from build123d import *

# Parameters (mm, degrees)
F0_W     = 152.4
F0_H     = 76.2
F1_DEPTH = 19.05
F2_SIZE  = 19.04999
F3_W     = 152.4
F3_H     = 76.2
F4_DEPTH = 10.16
F5_T     = -2.032
F6_R     = 5.08


# Not quite as in the source:
# - a fillet or chamfer is up to 0.001 mm smaller than in the source, because OpenCascade refuses the exact size


with BuildPart() as f1:
    # F0 (on Top) → F1 (new body)
    with BuildSketch(Plane.XY):
        with Locations((-76.2, -38.1)):
            Rectangle(F0_W, F0_H)
    extrude(amount=F1_DEPTH)

    # F2 (size 19.05 in the source; OpenCascade refuses exactly that, so slightly less here)
    f2_edges = [f1.edges().sort_by_distance(p)[0] for p in [
        (0, -38.1, 19.05),
        (-76.2, 0, 19.05),
        (-152.4, -38.1, 19.05),
        (-76.2, -76.2, 19.05),
    ]]
    chamfer(f2_edges, length=F2_SIZE)

    # F3 (on face) → F4 (join)
    with BuildSketch(Plane(origin=(0, 0, 0), x_dir=(1, 0, 0), z_dir=(0, 0, -1))):
        with Locations((-76.2, 38.1)):
            Rectangle(F3_W, F3_H)
    extrude(amount=F4_DEPTH)

    # F5
    f5_openings = [f1.faces().sort_by_distance(p)[0] for p in [
        (-76.2, -38.1, -10.16),
    ]]
    offset(amount=F5_T, openings=f5_openings)

    # F6
    f6_edges = [f1.edges().sort_by_distance(p)[0] for p in [
        (0, 0, -5.08),
        (-152.4, 0, -5.08),
        (-152.4, -76.2, -5.08),
        (0, -76.2, -5.08),
    ]]
    fillet(f6_edges, radius=F6_R)


solid = f1.part
Can you work these out from the model? Positions are in its coordinate system, mm. A direction names the side the tool comes from. Give positions to 0.01 mm unless a question says otherwise; leave off trailing zeros. Order: outer loops, then holes, each group sorted by start corner. A loop starts at its lowest first (then second) coordinate and runs counter-clockwise, first axis right, second up. Notation, with made-up numbers: M -34,0.25 L -12,0.25 A15 cw -12,17.25 Z; hole C -7,-3 d5. An arc over 180 degrees is marked long. One line per item, written item: value.
Item 1: If we section it at A-A on z = -8: Write out the boundary of the cut face in (x, y).
Verdict:
outline: M -152.4,-71.12 A5.08 ccw -147.32,-76.2 L -5.08,-76.2 A5.08 ccw 0,-71.12 L 0,-5.08 A5.08 ccw -5.08,0 L -147.32,0 A5.08 ccw -152.4,-5.08 Z; hole M -150.37,-74.17 L -2.03,-74.17 L -2.03,-2.03 L -150.37,-2.03 Z
Item 2: If we section it at B-B on x = -63.5: Write out the boundary of the cut face in (y, z).
Verdict:
outline: M -76.2,-10.16 L -74.17,-10.16 L -74.17,-0.84 L -56.31,17.02 L -19.89,17.02 L -2.03,-0.84 L -2.03,-10.16 L 0,-10.16 L 0,0 L -19.05,19.05 L -57.15,19.05 L -76.2,0 Z
Item 3: For pin 1 (4 mm diameter, centred on x = -62.5, z = 9.5, fed in from +Y); pin 2 (2 mm diameter, centred on x = -33.5, z = 9, fed in from -Y); pin 3 (10 mm diameter, centred on y = -30.5, z = 9, fed in from +X), each with a flat end and sliding along its axis, tell me the tip position at first contact or that it passes through.
Verdict:
pin 1: y = -7.5
pin 2: y = -68.2
pin 3: x = -4
Item 4: If we section it at D-D on z = 13: Write out the boundary of the cut face in (x, y).
Verdict:
outline: M -139.4,-63.2 L -13,-63.2 L -13,-13 L -139.4,-13 Z; hole M -136.53,-60.33 L -15.87,-60.33 L -15.87,-15.87 L -136.53,-15.87 Z
Item 5: If we mould it in two halves opening along X, with no side actions, what happens to faces 1 (the face through (-1.528, -1.449, -4.418)), 2 (the face through (-150.368, -38, -5)), 3 (the face through (-152.4, -38, -5))? For each: pulls with the +X half, pulls with the -X half, needs draft (parallel to the pull), parting line crosses it, or undercut.
Verdict:
face 1: pulls with the +X half
face 2: undercut
face 3: pulls with the -X half
Item 6: If we section it at C-C on y = -31: Write out the boundary of the cut face in (x, z).
Verdict:
outline: M -152.4,-10.16 L -150.37,-10.16 L -150.37,-0.84 L -132.51,17.02 L -19.89,17.02 L -2.03,-0.84 L -2.03,-10.16 L 0,-10.16 L 0,0 L -19.05,19.05 L -133.35,19.05 L -152.4,0 Z
Item 7: Please list where these lines run through material, in increasing order: line 1 (X direction, y = -46.5, z = -3); line 2 (Y direction, x = -40, z = -3.75); line 3 (X direction, y = -35, z = 16.5).
Verdict:
line 1: -152.4 to -150.37, -2.03 to 0
line 2: -76.2 to -74.17, -2.03 to 0
line 3: -135.9 to -133.03, -19.37 to -16.5
Item 8: For faces 4 (the face through (-77, -75, -10.16)), 5 (the face through (-2.032, -38, -5)), which set-ups out of +Z, -Z, +X, -X, +Y, -Y let a thin tool reach every point of the face, with its end or its side?
Verdict:
face 4: -Z, +X, -X, +Y, -Y
face 5: -Z
